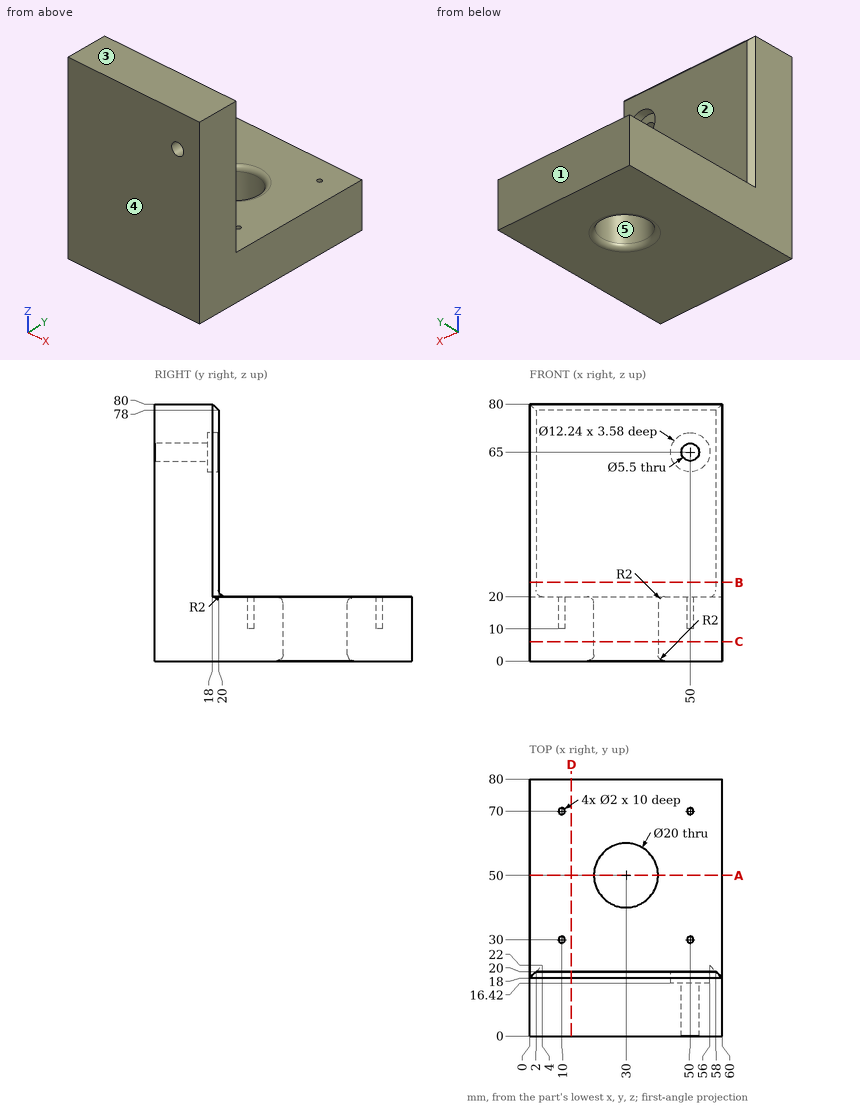
Study the drawing (mm; zero at the part's minimum x, y, z) and answer. A direction names the side the tool comes from. Round coordinates to 2 decimals unless told otherwise and drop trailing zeros. Write each loop counter-clockwise with the first axis right and the second up, starting at its lowest first coordinate (ties: lowest second). Pieces come first, ordered by that corner, then holes. Notation, with made-up numbers: (64.5, 72) -> (123.5, 72) arc R9 cw to (123.5, 81) -> close; hole circle Ø8 at (61, 0.25). An arc over 180 degrees is marked (long way). Write each question's results on one line, items separated by ' | '.
Item 1: A cutting plane is placed at C-C, the plane z = 6. Determine the outline of the cut face in (x, y), plus the area to 3 significant figures.
Result set:
outline: (0, 0) -> (60, 0) -> (60, 80) -> (0, 80) -> close; hole circle Ø20 at (30, 50) | area: 4,490 mm^2
Item 2: Which of the six approach directions +Z, -Z, +X, -X, +Y, -Y give full straight-line access (tool end or side, diameter ignored) to the marked faces 1 and 2?
Result set:
face 1: +Z, -Z, +X, -X, +Y | face 2: +Z, +X, -X, +Y
Item 3: Flat-ended cylindrical pins translate along their axes: P1, Ø6.5, axis at x = 50, z = 65, coming from the +Y side; P2, Ø5, axis at x = 29, z = 24.5, coming from the +Y side; P3, Ø2.5, axis at x = 10, y = 30, coming from the +Z side; P4, Ø16, axis at x = 30, y = 50, coming from the -Z side. Find the tip coordinate at first contact, or state that the pin passes through.
Result set:
P1: y = 16.42 | P2: y = 20 | P3: z = 20 | P4: through
Item 4: Find the intervals of material crossed by line 1 along Y through (x, z) = (10, 15.25); line 2 along Y through (x, z) = (30, 13); line 3 along Y through (x, z) = (7, 67), in increasing order. Write a range as [from, to].
Result set:
line 1: [0, 29], [31, 69], [71, 80] | line 2: [0, 40], [60, 80] | line 3: [0, 20]
Item 5: A cutting plane is placed at D-D, the plane x = 13. Determine the outline of the cut face in (y, z), plus the area to 3 significant figures.
Result set:
outline: (0, 0) -> (80, 0) -> (80, 20) -> (22, 20) arc R2 cw to (20, 22) -> (20, 78) -> (18, 80) -> (0, 80) -> close | area: 2,800 mm^2
Item 6: The mould has two halves that part along Y. Classify the marked faces 3, 4 and 5: +Y half, -Y half, draft (parallel to the pull), parting line (faces both ways), or undercut.
Result set:
face 3: draft | face 4: -Y half | face 5: undercut
Item 7: A cutting plane is placed at B-B, the plane z = 24.5. Determine the outline of the cut face in (x, y).
Result set:
outline: (0, 0) -> (60, 0) -> (60, 18) -> (58, 20) -> (2, 20) -> (0, 18) -> close
Item 8: A cutting plane is placed at A-A, the plane y = 50. Determine the outline of the cut face in (x, z), plus the area to 3 significant figures.
Result set:
outline: (0, 0) -> (18, 0) arc R2 ccw to (20, 2) -> (20, 18) arc R2 ccw to (18, 20) -> (0, 20) -> close; (40, 2) arc R2 ccw to (42, 0) -> (60, 0) -> (60, 20) -> (42, 20) arc R2 ccw to (40, 18) -> close | area: 797 mm^2
